Source: CAD feature listing. Evaluate the final solid. Frame: model axes, mm. Face numbers are marked on the shaded views. A direction names the side the tool comes from. Coordinates: 2 decimals unless noted, no trailing zeros. Write each loop counter-clockwise with the first axis right and the second up, starting at its lowest first coordinate (ties: lowest second). Pieces come first, ordered by that corner, then holes. Notation, with made-up numbers: M -1.5,62 L 13.5,62 A27 ccw 13.5,87 Z; hole C 66.25,71 d3. An arc over 180 degrees is marked long. One line per item, written item: value. Start each with the question number.
Item 1: Cut plane D-D, the plane y = 15. Output: boundary loops of the cut face in (x, z), then the cut area to 3 significant figures.
Item 2: Cut plane B-B, the plane x = 12.25. Output: boundary loops of the cut face in (y, z), then the cut area to 3 significant figures.
Item 3: Cut plane A-A, the plane y = -18. Output: boundary loops of the cut face in (x, z), then the cut area to 3 significant figures.
Item 4: Set-up query: the marked faces 5 and 6. Return all of +Z, -Z, +X, -X, +Y, -Y with unobstructed straight access to the full face (end or side cutting, diameter ignored); none if empty.
Item 5: Cut plane C-C, the plane z = -19.5. Output: boundary loops of the cut face in (x, y).
Item 6: Ray query, L1, parallel to Z at x = 8.75, y = -18; L2, parallel to Z at x = 8.25, y = 20; L3, parallel to Y at x = 11, z = 5. Return the intervals inside material, ascending. Write a range as from..to.
Item 7: Pin query (flat end, axial travel): P1, Ø6.5, axis at y = 20, z = 23, coming from the -X side; P2, Ø1, axis at x = 2.5, y = -1.5, coming from the -Z side; P3, Ø4.5, axis at x = 5.5, y = -22.5, coming from the -Z side; P4, Ø3, axis at x = 5.5, y = -19.5, coming from the -Z side. Return the tip coordinate at first contact, or that it passes through.
Item 8: Mould query, pull axis Z, two halves, no side actions, for the marked faces 1, 2, 3 and 4. Classes: released by +Z, released by -Z, zero draft, split by the parting line, or undercut.
```python
from build123d import *

# Parameters (mm, degrees)
F0_R     = 2
F0_R_2   = 16
F0_R_3   = 12
F1_DEPTH = 15


with BuildPart() as f1:
    # F0 (on Right) → F1 (new body)
    with BuildSketch(Plane.YZ):
        with BuildLine():
            Line((0, 27.04), (-25, 27.04))
            Line((-25, 27.04), (-25, 7.04))
            Line((-25, 7.04), (-21, 7.04))
            ThreePointArc((-21, 7.04), (-20.163638, 6.588177), (-20.08305, 5.640997))
            ThreePointArc((-20.08305, 5.640997), (-21.879632, -4.088083), (-19.211664, -13.615132))
            ThreePointArc((-19.211664, -13.615132), (-18.979502, -14.807582), (-19.480274, -15.914409))
            Line((-19.480274, -15.914409), (-20.600008, -17.156934))
            ThreePointArc((-20.600008, -17.156934), (-20.343066, -22.100008), (-15.399992, -21.843066))
            Line((-15.399992, -21.843066), (-15.041526, -21.44529))
            ThreePointArc((-15.041526, -21.44529), (-13.789573, -20.797894), (-12.421526, -21.136943))
            ThreePointArc((-12.421526, -21.136943), (-6.504182, -24.011949), (0, -25))
            ThreePointArc((0, -25), (18.034689, -17.736076), (26, 0))
            ThreePointArc((26, 0), (24.875659, 8.651645), (20.954714, 16.445315))
            ThreePointArc((20.954714, 16.445315), (20.567821, 17.729828), (21.079657, 18.969861))
            Line((21.079657, 18.969861), (22.600008, 20.656934))
            ThreePointArc((22.600008, 20.656934), (22.343066, 25.600008), (17.399992, 25.343066))
            Line((17.399992, 25.343066), (15.917898, 23.698445))
            ThreePointArc((15.917898, 23.698445), (14.727343, 23.05924), (13.402045, 23.32304))
            ThreePointArc((13.402045, 23.32304), (6.953967, 26.093547), (0, 27.04))
        make_face()
        with Locations((-18, -19.5)):
            Circle(F0_R, mode=Mode.SUBTRACT)
        Circle(F0_R_2, mode=Mode.SUBTRACT)
        with Locations((20, 23)):
            Circle(F0_R, mode=Mode.SUBTRACT)
        Circle(F0_R_2)
        Circle(F0_R_3, mode=Mode.SUBTRACT)
        Circle(F0_R_3)
    extrude(amount=F1_DEPTH)


solid = f1.part
```
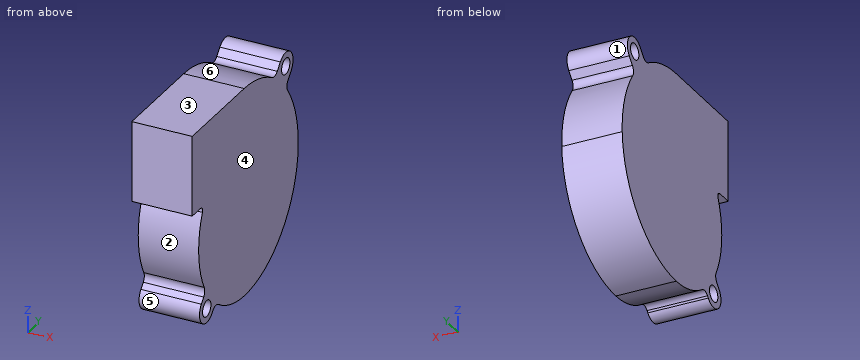
From the geometry:
1. outline: M 0,-20.24 L 15,-20.24 L 15,23.12 L 0,23.12 Z
1. area: 650 mm²
2. outline: M -25,7.04 L -21,7.04 A1 cw -20.08,5.64 A21.9 ccw -19.21,-13.62 A2 cw -19.48,-15.91 L -20.6,-17.16 A3.5 ccw -15.4,-21.84 L -15.04,-21.45 A2 cw -12.42,-21.14 A21.9 ccw 0,-25 A26.02 ccw 26,0 A26.02 ccw 20.95,16.45 A2 cw 21.08,18.97 L 22.6,20.66 A3.5 ccw 17.4,25.34 L 15.92,23.7 A2 cw 13.4,23.32 A26.02 ccw 0,27.04 L -25,27.04 Z; hole C -18,-19.5 d4; hole C 20,23 d4
2. area: 2,210 mm²
3. outline: M 0,-23 L 15,-23 L 15,-21.5 L 0,-21.5 Z; M 0,-17.5 L 15,-17.5 L 15,27.04 L 0,27.04 Z
3. area: 691 mm²
4. face 5: +X, -X
4. face 6: +Z, +X, -X
5. outline: M 0,-21.5 L 15,-21.5 L 15,-20 L 0,-20 Z; M 0,-16 L 15,-16 L 15,16 L 0,16 Z
6. L1: z = -23..-21.5, -17.5..27.04
6. L2: z = -15.62..21, 25..26.5
6. L3: y = -20.35..25.71
7. P1: stops at x = 0
7. P2: stops at z = -24.98
7. P3: stops at z = -22.18
7. P4: stops at z = -23
8. face 1: undercut
8. face 2: undercut
8. face 3: released by +Z
8. face 4: zero draft
